Part print with two shaded views. Sizes in mm from the minimum x, y, z corner. Give positions to 0.01 mm unless a question says otherwise; leave off trailing zeros. Order: outer loops, then holes, each group sorted by start corner. A loop starts at its lowest first (then second) coordinate and runs counter-clockwise, first axis right, second up. Notation, with made-up numbers: M 61.5,27.25 L 71.5,27.25 A10 cw 71.5,41.25 Z; hole C 29.25,69.5 d5. An arc over 180 degrees is marked long. Answer as CSV lines item,"result".
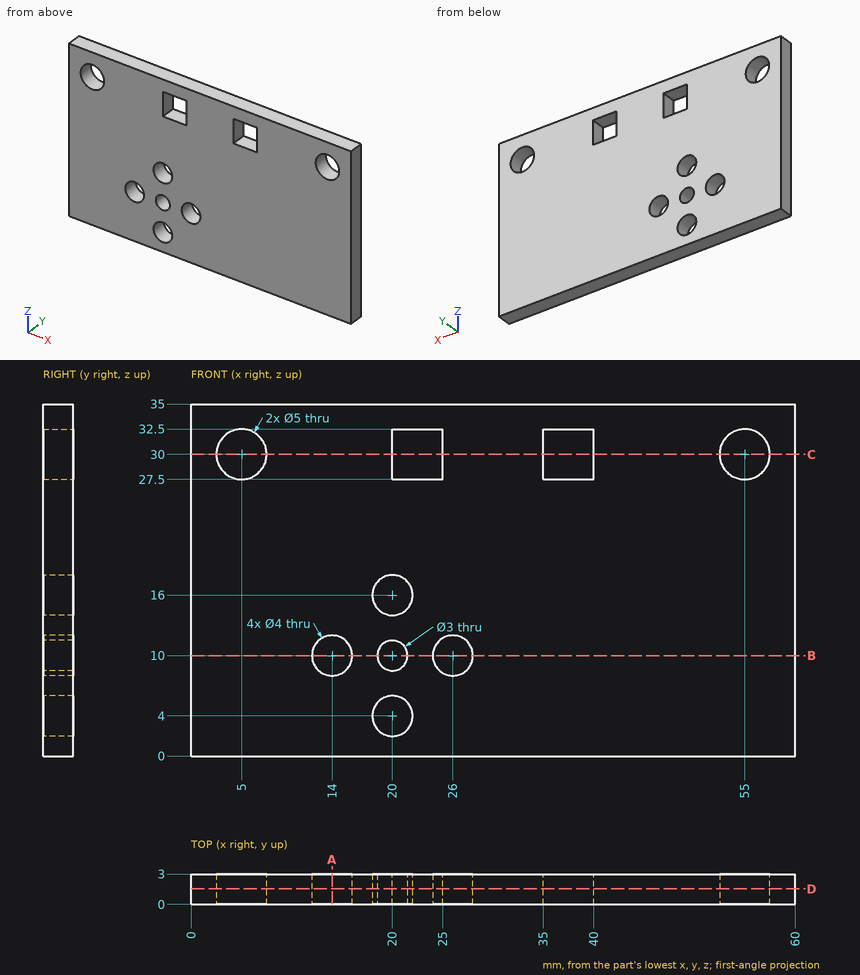
Item 1: Band-saw the part on A-A (x = 14). Give the cut face in (y, z).
Geometry says:
outline,"M 0,0 L 3,0 L 3,8 L 0,8 Z; M 0,12 L 3,12 L 3,35 L 0,35 Z"
Item 2: Band-saw the part on C-C (z = 30). Give the cut face in (x, y).
Geometry says:
outline,"M 0,0 L 2.5,0 L 2.5,3 L 0,3 Z; M 7.5,0 L 20,0 L 20,3 L 7.5,3 Z; M 25,0 L 35,0 L 35,3 L 25,3 Z; M 40,0 L 52.5,0 L 52.5,3 L 40,3 Z; M 57.5,0 L 60,0 L 60,3 L 57.5,3 Z"
Item 3: Drop a flat-ended pin along its axis: pin 1 (3 mm diameter, centred on x = 55, z = 30, fed in from +Y). Give the stop position or say it passes through.
Geometry says:
pin 1,"passes through"
Item 4: Band-saw the part on D-D (y = 1.55). State how many separate pieces and enclosed holes the cut face has, and give its area (3 significant figures).
Geometry says:
separate pieces,"1"
enclosed holes,"9"
area,"1,950 mm2"
Item 5: Band-saw the part on B-B (z = 10). Give the cut face in (x, y), and give its area (3 significant figures).
Geometry says:
outline,"M 0,0 L 12,0 L 12,3 L 0,3 Z; M 16,0 L 18.5,0 L 18.5,3 L 16,3 Z; M 21.5,0 L 24,0 L 24,3 L 21.5,3 Z; M 28,0 L 60,0 L 60,3 L 28,3 Z"
area,"147 mm2"
Item 6: Probe line 1 along X through (y, z) = (1.9, 10.5); line 2 along Z through (x, y) = (14, 1.8); line 3 along Z through (x, y) = (5, 0.7). List the from-to ranges inside material, lowest first. Write a range as from..to.
Geometry says:
line 1,"x = 0..12.06, 15.94..18.59, 21.41..24.06, 27.94..60"
line 2,"z = 0..8, 12..35"
line 3,"z = 0..27.5, 32.5..35"
